Check sheet for the modelled part. Datum: model origin and axes. Units: mm. A direction names the side the tool comes from. Round coordinates to 2 decimals unless told otherwise and drop trailing zeros. Order: outer loops, then holes, each group sorted by start corner. A loop starts at its lowest first (then second) coordinate and runs counter-clockwise, first axis right, second up. Notation, with made-up numbers: (34.5, 16.5) -> (75.5, 16.5) arc R19 ccw to (75.5, 47.5) -> close; hole circle Ø7 at (-0.75, 89.5). An arc over 180 degrees is marked (long way). Use CSV: the item, a comma, the result in double quotes.
```python
from build123d import *

# Parameters (mm, degrees)
EXTRUDE_2_DEPTH           = 3
SKETCH_4_R                = 2.25
SKETCH_4_R_2              = 2.5
CUT_EXTRUDE_2_DEPTH       = 96.402519291
SKETCH_6_R                = 3.5
CUT_EXTRUDE_3_DEPTH       = 96.402519291
SKETCH_7_R                = 3.5
CUT_EXTRUDE_4_DEPTH       = 96.402519291
CUT_EXTRUDE_5_DEPTH       = 96.402519291
EXTRUDE_4_DEPTH           = 15
EXTRUDE_5_DEPTH           = 3
SKETCH_11_R               = 4.1
CUT_EXTRUDE_6_DEPTH       = 3
SKETCH_13_R               = 3.5
EXTRUDE_6_DEPTH           = 3
SKETCH_14_R               = 2.05
EXTRUDE_7_DEPTH           = 5
EXTRUDE_START             = -5
SKETCH_15_R               = 4
SKETCH_15_R_2             = 2.05
EXTRUDE_8_DEPTH           = 5
CUT_EXTRUDE_7_DEPTH       = 96.878259721
SKETCH_18_R               = 1.397318861
CUT_EXTRUDE_8_DEPTH       = 144.753442506
CUT_EXTRUDE_9_DEPTH       = 97.527927136
CUT_EXTRUDE_9_DEPTH_BACK  = 97.527927136
CUT_EXTRUDE_11_DEPTH      = 110.140706759
CUT_EXTRUDE_11_DEPTH_BACK = 110.140706759
SKETCH_20_W               = 92.736362136
SKETCH_20_H               = 2.6
SKETCH_20_H_2             = 2.5


with BuildPart() as part:
    # 草图2 → 凸台-拉伸2 (new body)
    with BuildSketch(Plane(origin=(0, 0, 0), x_dir=(1, 0, 0), z_dir=(0, 1, 0))):
        with BuildLine():
            Line((-58.569449541, 23.337085947), (32.740581269, -53.879999426))
            ThreePointArc((32.740581269, -53.879999426), (53.033008589, -53.033008589), (53.879999426, -32.740581269))
            Line((53.879999426, -32.740581269), (-23.337085947, 58.569449541))
            ThreePointArc((-23.337085947, 58.569449541), (-60.104076401, 60.104076401), (-58.569449541, 23.337085947))
        make_face()
    extrude(amount=EXTRUDE_2_DEPTH)

    # 草图4 → 切除-拉伸2 (cut, through all)
    with BuildSketch(Plane(origin=(0, 3, 0), x_dir=(1, 0, 0), z_dir=(0, 1, 0))):
        with Locations(Location((-42.426406871, 42.426406871, 0), (0, 0, 270))):
            Circle(SKETCH_4_R)
        with Locations(Location((42.426406871, -42.426406871, 0), (0, 0, 270))):
            Circle(SKETCH_4_R_2)
    extrude(amount=-CUT_EXTRUDE_2_DEPTH, mode=Mode.SUBTRACT)

    # 草图6 → 切除-拉伸3 (cut, through all)
    with BuildSketch(Plane(origin=(0, 3, 0), x_dir=(1, 0, 0), z_dir=(0, 1, 0))):
        with Locations(Location((-42.426406871, 42.426406871, 0), (0, 0, 270))):
            Circle(SKETCH_6_R)
    extrude(amount=-CUT_EXTRUDE_3_DEPTH, mode=Mode.SUBTRACT)

    # 草图7 → 切除-拉伸4 (cut, through all)
    with BuildSketch(Plane(origin=(0, 3, 0), x_dir=(1, 0, 0), z_dir=(0, 1, 0))):
        with Locations(Location((42.426406871, -42.426406871, 0), (0, 0, 270))):
            Circle(SKETCH_7_R)
    extrude(amount=-CUT_EXTRUDE_4_DEPTH, mode=Mode.SUBTRACT)

    # 草图8 → 切除-拉伸5 (cut, through all)
    with BuildSketch(Plane(origin=(0, 3, 0), x_dir=(1, 0, 0), z_dir=(0, 1, 0))):
        Polygon((33.626672858, -22.564710472), (-15.702999665, 25.870376375), (-26.891422763, 12.98046534), (25.218843822, -32.251166492), align=None)
    extrude(amount=-CUT_EXTRUDE_5_DEPTH, mode=Mode.SUBTRACT)

    # 草图9 → 凸台-拉伸4 (add)
    with BuildSketch(Plane(origin=(0, 3, 0), x_dir=(1, 0, 0), z_dir=(0, 1, 0))):
        with BuildLine():
            ThreePointArc((-17.960284018, 47.565359346), (-19.96440182, 53.401757848), (-23.337085947, 58.569449541))
            ThreePointArc((-23.337085947, 58.569449541), (-60.104076401, 60.104076401), (-58.569449541, 23.337085947))
            ThreePointArc((-58.569449541, 23.337085947), (-53.401757848, 19.96440182), (-47.565359346, 17.960284018))
            Line((-47.565359346, 17.960284018), (-56.632284421, 25.627804458))
            ThreePointArc((-56.632284421, 25.627804458), (-57.982756057, 57.982756057), (-25.627804458, 56.632284421))
            Line((-25.627804458, 56.632284421), (-17.960284018, 47.565359346))
        make_face()
        with BuildLine():
            Line((53.879999426, -32.740581269), (-23.337085947, 58.569449541))
            ThreePointArc((-23.337085947, 58.569449541), (-19.96440182, 53.401757848), (-17.960284018, 47.565359346))
            Line((-17.960284018, 47.565359346), (45.777785554, -27.805590857))
            ThreePointArc((45.777785554, -27.805590857), (50.229311839, -29.615681908), (53.879999426, -32.740581269))
        make_face()
        with BuildLine():
            ThreePointArc((-47.565359346, 17.960284018), (-53.401757848, 19.96440182), (-58.569449541, 23.337085947))
            Line((-58.569449541, 23.337085947), (32.740581269, -53.879999426))
            ThreePointArc((32.740581269, -53.879999426), (29.615681908, -50.229311839), (27.805590857, -45.777785554))
            Line((27.805590857, -45.777785554), (-47.565359346, 17.960284018))
        make_face()
        with BuildLine():
            ThreePointArc((57.426406871, -42.426406871), (56.511929373, -37.26907657), (53.879999426, -32.740581269))
            ThreePointArc((53.879999426, -32.740581269), (50.229311839, -29.615681908), (45.777785554, -27.805590857))
            Line((45.777785554, -27.805590857), (51.589280915, -34.67774639))
            ThreePointArc((51.589280915, -34.67774639), (53.694824873, -38.30054263), (54.426406871, -42.426406871))
            ThreePointArc((54.426406871, -42.426406871), (47.47695507, -53.311808237), (34.67774639, -51.589280915))
            Line((34.67774639, -51.589280915), (27.805590857, -45.777785554))
            ThreePointArc((27.805590857, -45.777785554), (29.615681908, -50.229311839), (32.740581269, -53.879999426))
            ThreePointArc((32.740581269, -53.879999426), (48.73959212, -56.033158578), (57.426406871, -42.426406871))
        make_face()
    extrude(amount=EXTRUDE_4_DEPTH)

    # 草图10 → 凸台-拉伸5 (add)
    with BuildSketch(Plane(origin=(0, 3, 0), x_dir=(1, 0, 0), z_dir=(0, 1, 0))):
        Polygon((10.528753113, -10.528753113), (-20.427450775, 20.427450775), (-26.891422763, 12.98046534), (25.218843822, -32.251166492), (28.486536718, -28.486536718), align=None)
        Polygon((-15.702999665, 25.870376375), (-20.427450775, 20.427450775), (10.528753113, -10.528753113), (28.486536718, -28.486536718), (33.626672858, -22.564710472), align=None)
    extrude(amount=-EXTRUDE_5_DEPTH)

    # 草图11 → 切除-拉伸6 (cut)
    with BuildSketch(Plane(origin=(0, 3, 0), x_dir=(1, 0, 0), z_dir=(0, 1, 0))):
        with Locations(Location((-21.213203436, 21.213203436, 0), (0, 0, 270))):
            Circle(SKETCH_11_R)
    extrude(amount=-CUT_EXTRUDE_6_DEPTH, mode=Mode.SUBTRACT)

    # 草图13 → 凸台-拉伸6 (add)
    with BuildSketch(Plane(origin=(0, 3, 0), x_dir=(1, 0, 0), z_dir=(0, 1, 0))):
        with Locations((-42.426406871, 42.426406871)):
            Circle(SKETCH_13_R)
    extrude(amount=-EXTRUDE_6_DEPTH)

    # 草图14 → 凸台-拉伸7 (add)
    with BuildSketch(Plane(origin=(0, 3, 0), x_dir=(1, 0, 0), z_dir=(0, 1, 0))):
        with Locations(Location((-42.426406871, 42.426406871, 0), (0, 0, 270))):
            Circle(SKETCH_14_R)
    extrude(amount=EXTRUDE_7_DEPTH)

    # 草图15 → 凸台-拉伸8 (add)
    with BuildSketch(Plane(origin=(0, 8, 0), x_dir=(1, 0, 0), z_dir=(0, 1, 0)).offset(EXTRUDE_START)):
        with Locations(Location((-42.426406871, 42.426406871, 0), (0, 0, 270))):
            Circle(SKETCH_15_R)
        with Locations((-42.426406871, 42.426406871)):
            Circle(SKETCH_15_R_2, mode=Mode.SUBTRACT)
    extrude(amount=EXTRUDE_8_DEPTH)

    # 草图17 → 切除-拉伸7 (cut, through all)
    with BuildSketch(Plane(origin=(0, 8, 0), x_dir=(1, 0, 0), z_dir=(0, 1, 0))):
        with BuildLine():
            Line((-42.409215342, 44.476334785), (-43.439595085, 43.532503451))
            Line((-43.439595085, 43.532503451), (-44.469974827, 42.588672118))
            ThreePointArc((-44.469974827, 42.588672118), (-42.507603209, 40.378015513), (-40.376406871, 42.426406871))
            ThreePointArc((-40.376406871, 42.426406871), (-40.970772536, 43.869884853), (-42.409215342, 44.476334785))
        make_face()
    extrude(amount=-CUT_EXTRUDE_7_DEPTH, mode=Mode.SUBTRACT)

    # 草图18 → 切除-拉伸8 (cut, through all)
    with BuildSketch(Plane(origin=(-41.501827845, 0, -45.307504805), x_dir=(0.7373977200215518, 0, -0.6754588088899406), z_dir=(0.6754588088899406, 0, 0.7373977200215518))):
        with Locations((-2.627845445, 4.953208644)):
            Circle(SKETCH_18_R)
    extrude(amount=-CUT_EXTRUDE_8_DEPTH, mode=Mode.SUBTRACT)

    # 草图19 → 切除-拉伸9 (cut, two sides: drawn at the far end of the back side and taken through both)
    with BuildSketch(Plane(origin=(0, 3, 0), x_dir=(1, 0, 0), z_dir=(0, 1, 0)).offset(-CUT_EXTRUDE_9_DEPTH_BACK)):
        with BuildLine():
            Line((-66.29326799, 34.985107232), (-63.429244656, 35.878063189))
            ThreePointArc((-63.429244656, 35.878063189), (-57.900931168, 58.064152802), (-35.65805893, 63.35938244))
            Line((-35.65805893, 63.35938244), (-34.735102393, 66.213879108))
            ThreePointArc((-34.735102393, 66.213879108), (-60.011093572, 60.196572701), (-66.29326799, 34.985107232))
        make_face()
    extrude(amount=CUT_EXTRUDE_9_DEPTH + CUT_EXTRUDE_9_DEPTH_BACK, mode=Mode.SUBTRACT)

    # 草图20 → 切除-拉伸11 (cut, two sides: drawn at the far end of the back side and taken through both)
    with BuildSketch(Plane(origin=(-12.914434136, 0, 15.27145674), x_dir=(0.7635728369858691, 0, 0.6457217067881111), z_dir=(-0.6457217067881111, 0, 0.7635728369858691)).offset(-CUT_EXTRUDE_11_DEPTH_BACK)):
        with Locations((13.423122648, 10.3)):
            Rectangle(SKETCH_20_W, SKETCH_20_H)
        with Locations((13.423122648, 7.75)):
            Rectangle(SKETCH_20_W, SKETCH_20_H_2)
    extrude(amount=CUT_EXTRUDE_11_DEPTH + CUT_EXTRUDE_11_DEPTH_BACK, mode=Mode.SUBTRACT)


solid = part.part
```
Q1. Sectioned sample at C-C, the plane x = 17. Enter the section's corners in (y, z).
Result sheet:
outline,"(0, -10.87) -> (6.5, -10.87) -> (6.5, -6.22) -> (3, -6.22) -> (3, 36.64) -> (6.5, 36.64) -> (6.5, 40.57) -> (0, 40.57) -> close; (11.6, -10.87) -> (18, -10.87) -> (18, -6.22) -> (11.6, -6.22) -> close; (11.6, 36.64) -> (18, 36.64) -> (18, 40.57) -> (11.6, 40.57) -> close"
Q2. Sectioned sample at D-D, the plane z = -14. Enter the section's corners in (x, y), then the cut area to 3 significant figures.
Result sheet:
outline,"(-47.53, 0) -> (14.35, 0) -> (14.35, 6.5) -> (10.42, 6.5) -> (10.42, 3) -> (-42.88, 3) -> (-42.88, 18) -> (-47.53, 18) -> close; (10.42, 11.6) -> (14.35, 11.6) -> (14.35, 18) -> (10.42, 18) -> close"
area,"294 mm^2"
Q3. Access from +Z, -Z, +X, -X, +Y, -Y to the whole of each face (thin tool, end or side, straight path). Record for faces 1 (the face through (-41.225, 5.465, -38.611)), 2 (the face through (-44.41, 6.34, -44.32)), 3 (the face through (-44.1, 8, -43.4)).
Result sheet:
face 1,"+Y"
face 2,"none"
face 3,"-Z, -X, +Y"
Q4. Mould release check, pull along X, two halves, no side actions. Record for faces 4 (the face through (21, 11.6, -4)), 5 (the face through (-60.713, 10.395, -30.196)), 6 (the face through (-30.243, 10.395, -60.745)): pulls with the +X half, pulls with the -X half, needs draft (parallel to the pull), parting line crosses it, or undercut.
Result sheet:
face 4,"needs draft"
face 5,"undercut"
face 6,"pulls with the -X half"
Q5. Sectioned sample at A-A, the plane y = 16.25. Enter the section's corners in (x, z), then the cut area to 3 significant figures.
Result sheet:
outline,"(-66.29, -34.99) -> (-63.43, -35.88) arc R22 cw to (-56.63, -25.63) -> (34.68, 51.59) arc R12 cw to (51.59, 34.68) -> (-25.63, -56.63) arc R22 cw to (-35.66, -63.36) -> (-34.74, -66.21) arc R25 ccw to (-23.34, -58.57) -> (53.88, 32.74) arc R15 ccw to (32.74, 53.88) -> (-58.57, -23.34) arc R25 ccw to start"
area,"917 mm^2"
Q6. Go/stop test with flat-tipped pins: pin 1 (1 mm diameter, centred on x = -23, y = 11.5, fed in from +Z); pin 2 (5 mm diameter, centred on y = 5.5, z = 1.5, fed in from +X); pin 3 (1.5 mm diameter, centred on x = 22.5, y = 15.5, fed in from -Z). Record where each tip stops, or that it passes through.
Result sheet:
pin 1,"stops at z = 7.16"
pin 2,"stops at x = 29.58"
pin 3,"stops at z = -5.25"
Q7. Scan lines: L1, parallel to Y at x = 39, z = 27; L2, parallel to Z at x = -16, y = 14.5; L3, parallel to X at y = 5, z = -30.5. Record each from-to range of solid material in increasing order.
Result sheet:
L1,"y = 0 to 3"
L2,"z = -49.89 to -45.25, 8.73 to 12.66"
L3,"x = -64.4 to -60.91, -3.53 to 0.4"
Q8. Sectioned sample at B-B, the plane z = 10. Enter the section's corners in (x, y), then the cut area to 3 significant figures.
Result sheet:
outline,"(-19.15, 0) -> (34.65, 0) -> (34.65, 6.5) -> (30.72, 6.5) -> (30.72, 3) -> (-14.5, 3) -> (-14.5, 6.5) -> (-19.15, 6.5) -> close; (-19.15, 11.6) -> (-14.5, 11.6) -> (-14.5, 18) -> (-19.15, 18) -> close; (30.72, 11.6) -> (34.65, 11.6) -> (34.65, 18) -> (30.72, 18) -> close"
area,"246 mm^2"
